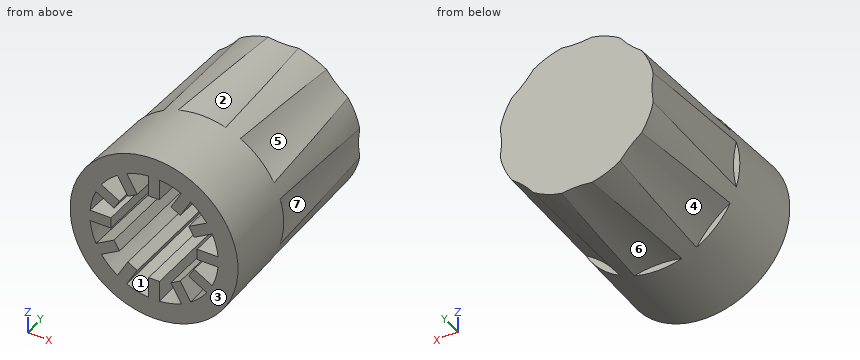
from build123d import *

# Parameters (mm, degrees)
SKETCH2_R           = 7.624300038
CUT_EXTRUDE1_DEPTH  = 10
CIRPATTERN1_COUNT   = 8
SKETCH3_W           = 1.605
SKETCH3_H           = 0.82
SKETCH3_W_2         = 0.82
SKETCH3_H_2         = 1.605
BOSS_EXTRUDE1_DEPTH = 14.88


with BuildPart() as part:
    # Sketch1 → Revolve1 (revolve)
    with BuildSketch(Plane.XY, mode=Mode.PRIVATE) as revolve1_sk:
        Polygon((-6.375, 0), (-5.92, 15.88), (0, 15.88), (0, 14.88), (-4.448652393, 14.88), (-4.875, 0), align=None)
    revolve(revolve1_sk.sketch.rotate(Axis((0, 0, 0), (0, 1, 0)), 270), axis=Axis((0, 0, 0), (0, 1, 0)))

    # Sketch2 → Cut-Extrude1 (cut)
    with BuildSketch(Plane(origin=(0, 15.88, 0), x_dir=(1, 0, 0), z_dir=(0, 1, 0))):
        with Locations((-13.344300038, 0)):
            Circle(SKETCH2_R)
    cut_extrude1 = extrude(amount=-CUT_EXTRUDE1_DEPTH, mode=Mode.SUBTRACT)

    # CirPattern1: Cut-Extrude1 ×8 about axis
    cirpattern1_axis = Axis((0, 0, 0), (0, 1, 0))
    for i in range(1, CIRPATTERN1_COUNT):
        add(cut_extrude1.rotate(cirpattern1_axis, i * 360 / CIRPATTERN1_COUNT), mode=Mode.SUBTRACT)

    # Sketch3 → Boss-Extrude1 (add)
    with BuildSketch(Plane.XZ.offset(-14.88)):
        with Locations((-4.0725, 0)):
            Rectangle(SKETCH3_W, SKETCH3_H)
        Polygon((-4.016873843, 2.792570416), (-2.62690307, 1.990070416), (-3.03690307, 1.279929584), (-4.426873843, 2.082429584), align=None)
        Polygon((-2.082429584, 4.426873843), (-1.279929584, 3.03690307), (-1.990070416, 2.62690307), (-2.792570416, 4.016873843), align=None)
        with Locations((0, 4.0725)):
            Rectangle(SKETCH3_W_2, SKETCH3_H_2)
        Polygon((2.792570416, 4.016873843), (1.990070416, 2.62690307), (1.279929584, 3.03690307), (2.082429584, 4.426873843), align=None)
        Polygon((4.426873843, 2.082429584), (3.03690307, 1.279929584), (2.62690307, 1.990070416), (4.016873843, 2.792570416), align=None)
        with Locations((4.0725, 0)):
            Rectangle(SKETCH3_W, SKETCH3_H)
        Polygon((4.016873843, -2.792570416), (2.62690307, -1.990070416), (3.03690307, -1.279929584), (4.426873843, -2.082429584), align=None)
        Polygon((2.082429584, -4.426873843), (1.279929584, -3.03690307), (1.990070416, -2.62690307), (2.792570416, -4.016873843), align=None)
        with Locations((0, -4.0725)):
            Rectangle(SKETCH3_W_2, SKETCH3_H_2)
        Polygon((-2.792570416, -4.016873843), (-1.990070416, -2.62690307), (-1.279929584, -3.03690307), (-2.082429584, -4.426873843), align=None)
        Polygon((-4.426873843, -2.082429584), (-3.03690307, -1.279929584), (-2.62690307, -1.990070416), (-4.016873843, -2.792570416), align=None)
    extrude(amount=BOSS_EXTRUDE1_DEPTH)


solid = part.part
Check sheet for the modelled part. Datum: model origin and axes. Units: mm. Face numbers are marked on the shaded views. A direction names the side the tool comes from. Give positions to 0.01 mm unless a question says otherwise; leave off trailing zeros. Loops run counter-clockwise (first coordinate to the right, second up) from the corner with the lowest first, then second, coordinate; pieces in that order, holes last. Notation, with made-up numbers: M 26,16 L 40,16 A16 ccw 40,35 Z; hole C 21,68.25 d11. An arc over 180 degrees is marked long. Use a Markdown table: item, result. Add a question column.
Q1. Scan lines: line 1 along X through (y, z) = (5.5, -1.5); line 2 along Z through (x, y) = (-1.75, 14); line 3 along Z through (x, y) = (0, 7.5). Record each from-to range of solid material in increasing order. Write a range as [from, to].
Q2. Mould release check, pull along Z, two halves, no side actions. Record for the marked faces 1, 2 and 3: pulls with the +Z half, pulls with the -Z half, needs draft (parallel to the pull), parting line crosses it, or undercut.
Q3. Sectioned sample at B-B, the plane x = 0. Record the cut outline in (y, z) (3 decimals).
Q4. Tool access check on the marked faces 4, 5, 6 and 7. Record the directions out of +Z, -Z, +X, -X, +Y, -Y that give a thin tool (end or side, any length) a straight path to the whole face; none if there is none.
Q5. Go/stop test with flat-tipped pins: pin 1 (1.3 mm diameter, centred on x = 4.5, z = 4, fed in from +Y); pin 2 (6 mm diameter, centred on y = 5, z = 4, fed in from -X); pin 3 (0.5 mm diameter, centred on x = -4.5, y = 7.5, fed in from -Z); pin 4 (0.5 mm diameter, centred on y = 8.5, z = 4, fed in from -X). Record where each tip stops, or that it passes through.
Q6. Sectioned sample at A-A, the plane z = 0. Record the cut outline in (x, y) (3 decimals), then the cut area to 3 significant figures.
Verdict:
| question | item | result |
|---|---|---|
| 1 | line 1 | [-6.03, -4.47], [-3.42, -2.91], [2.91, 3.42], [4.47, 6.03] |
| 1 | line 2 | [-5.71, -4.12], [-3.85, -2.77], [2.77, 3.85], [4.12, 5.71] |
| 1 | line 3 | [-5.72, -3.27], [3.27, 5.72] |
| 2 | face 1 | undercut |
| 2 | face 2 | pulls with the +Z half |
| 2 | face 3 | needs draft |
| 3 | outline | M 0,-6.375 L 5.88,-6.207 L 5.88,-5.72 L 15.88,-5.72 L 15.88,5.72 L 5.88,5.72 L 5.88,6.207 L 0,6.375 L 0,3.27 L 14.88,3.27 L 14.88,-3.27 L 0,-3.27 Z |
| 4 | face 4 | -Z, -X, +Y |
| 4 | face 5 | +Z, +X, +Y |
| 4 | face 6 | -Z, +Y |
| 4 | face 7 | +X, +Y |
| 5 | pin 1 | y = 15.88 |
| 5 | pin 2 | x = -6.16 |
| 5 | pin 3 | z = -3.85 |
| 5 | pin 4 | x = -4.36 |
| 6 | outline | M -6.375,0 L -3.27,0 L -3.27,14.88 L 3.27,14.88 L 3.27,0 L 6.375,0 L 6.207,5.88 L 5.72,5.88 L 5.72,15.88 L -5.72,15.88 L -5.72,5.88 L -6.207,5.88 Z |
| 6 | area | 91.1 mm^2 |
